Build history of the part. All positions in model axes, mm. A direction names the side the tool comes from. Coordinates: 2 decimals unless noted, no trailing zeros. Order: outer loops, then holes, each group sorted by start corner. A loop starts at its lowest first (then second) coordinate and runs counter-clockwise, first axis right, second up. Notation, with made-up numbers: M 43.25,-2.5 L 75.25,-2.5 A30 ccw 75.25,28.5 Z; hole C -2,0.5 d8. An arc over 180 degrees is marked long. Write item = value, one per line. Start each with the question number.
Q1. 3-axis set-ups, long thin cutter, end or side, ignore diameter. For faces 1 (the face through (25.3, 4, 2.4)), 2 (the face through (31.24, -2.03, 6.94)), 3 (the face through (0.488, 0.986, 30.696)): which of +Z, -Z, +X, -X, +Y, -Y reach the whole face in a straight line?
Q2. Band-saw the part on A-A on x = 0. Write the cut outline in (y, z), plus the area to 3 significant figures.
Q3. Band-saw the part on C-C on y = 4.5. Write the cut outline in (x, z).
Q4. Band-saw the part on B-B on z = 0. Write the cut outline in (x, y), plus the area to 3 significant figures.
Q5. Pin check, flat tips, straight feed: P1, Ø1.5, axis at y = -1, z = 9, coming from the +X side; P2, Ø7, axis at x = 0, z = 28.5, coming from the +Y side; P3, Ø4, axis at y = 0, z = -24, coming from the +X side; P4, Ø2.5, axis at x = 0, z = 28.5, coming from the +Y side. Stop position of each tip, or through.
Q6. Drill centre lines: probe 1 along X at (y, z) = (-2.5, 0); probe 2 along Y at (x, z) = (-18, 8); probe 3 along Z at (x, y) = (28.5, 3.95). Where is each one in solid material? Low to high.
Q7. Band-saw the part on D-D on z = -28.5. Write the cut outline in (x, y).
```python
from build123d import *

# Parameters (mm, degrees)
CBORE_FOR_M4_SHCS1_D           = 4.5
CBORE_FOR_M4_SHCS1_CBORE_D     = 8
CBORE_FOR_M4_SHCS1_CBORE_DEPTH = 4
M4X0_7_TAPPED_HOLE1_D          = 3.3
M4X0_7_TAPPED_HOLE1_DEPTH      = 8.1
M4X0_7_TAPPED_HOLE1_TIP        = 0.991420021
SKETCH7_R                      = 1.5
CUT_EXTRUDE1_DEPTH             = 52.884487084


with BuildPart() as part:
    # Sketch2 → Revolve1 (revolve)
    with BuildSketch(Plane.XY, mode=Mode.PRIVATE) as revolve1_sk:
        Polygon((0, 0), (32, 0), (32, -4), (36, -4), (36, 6), (0, 6), align=None)
    revolve(revolve1_sk.sketch.rotate(Axis((0, -990.217396251, 0), (0, 1, 0)), 90), axis=Axis((0, -990.217396251, 0), (0, 1, 0)))

    # CBORE for M4 SHCS1 (through all)
    with Locations(Plane(origin=(0, 6, 0), x_dir=(1, 0, 0), z_dir=(0, 1, 0))):
        with Locations((0, 28.5), (-28.5, 0), (28.5, 0), (0, -28.5)):
            CounterBoreHole(CBORE_FOR_M4_SHCS1_D / 2, CBORE_FOR_M4_SHCS1_CBORE_D / 2, CBORE_FOR_M4_SHCS1_CBORE_DEPTH)

    # M4x0.7 Tapped Hole1
    with Locations(Plane(origin=(0, 6, 0), x_dir=(1, 0, 0), z_dir=(0, 1, 0))):
        with Locations((-14.142135624, 14.142135624), (14.142135624, -14.142135624)):
            Hole(M4X0_7_TAPPED_HOLE1_D / 2, depth=M4X0_7_TAPPED_HOLE1_DEPTH)
            with Locations((0, 0, -(M4X0_7_TAPPED_HOLE1_DEPTH + M4X0_7_TAPPED_HOLE1_TIP / 2))):  # 118° drill point
                Cone(0, M4X0_7_TAPPED_HOLE1_D / 2, M4X0_7_TAPPED_HOLE1_TIP, mode=Mode.SUBTRACT)

    # Sketch7 → Cut-Extrude1 (cut, through all)
    with BuildSketch(Plane(origin=(0, 6, 0), x_dir=(1, 0, 0), z_dir=(0, 1, 0))):
        with Locations(Location((0, 0, 0), (0, 0, 270))):
            Circle(SKETCH7_R)
    extrude(amount=-CUT_EXTRUDE1_DEPTH, mode=Mode.SUBTRACT)


solid = part.part
```
Recorded:
q1.face_1 = +Y
q1.face_2 = -Y
q1.face_3 = +Y, -Y
q2.outline = M -4,-36 L 6,-36 L 6,-32.5 L 2,-32.5 L 2,-30.75 L 0,-30.75 L 0,-32 L -4,-32 Z; M -4,32 L 0,32 L 0,30.75 L 2,30.75 L 2,32.5 L 6,32.5 L 6,36 L -4,36 Z; M 0,-26.25 L 2,-26.25 L 2,-24.5 L 6,-24.5 L 6,-1.5 L 0,-1.5 Z; M 0,1.5 L 6,1.5 L 6,24.5 L 2,24.5 L 2,26.25 L 0,26.25 Z
q2.area = 364 mm2
q3.outline = C 0,0 d72; hole C -28.5,0 d8; hole C -14.14,-14.14 d3.3; hole C 0,-28.5 d8; hole C 0,28.5 d8; hole C 0,0 d3; hole C 14.14,14.14 d3.3; hole C 28.5,0 d8
q4.outline = M -36,-4 L -32,-4 L -32,0 L -30.75,0 L -30.75,2 L -32.5,2 L -32.5,6 L -36,6 Z; M -26.25,0 L -1.5,0 L -1.5,6 L -24.5,6 L -24.5,2 L -26.25,2 Z; M 1.5,0 L 26.25,0 L 26.25,2 L 24.5,2 L 24.5,6 L 1.5,6 Z; M 30.75,0 L 32,0 L 32,-4 L 36,-4 L 36,6 L 32.5,6 L 32.5,2 L 30.75,2 Z
q4.area = 364 mm2
q5.P1 = 35.04
q5.P2 = 2
q5.P3 = 28.5
q5.P4 = through
q6.probe_1 = -36 to -32, 32 to 36
q6.probe_2 = 0 to 6
q6.probe_3 = -21.99 to -4, 4 to 21.99
q7.outline = M -21.99,-4 L -14.55,-4 L -14.55,0 L -2.25,0 L -2.25,2 L -4,2 L -4,6 L -21.99,6 Z; M 2.25,0 L 14.55,0 L 14.55,-4 L 21.99,-4 L 21.99,6 L 4,6 L 4,2 L 2.25,2 Z
